For this review, use the dimensioned drawing (mm, ordinates from the lowest corner) and the shaded views. A direction names the side the tool comes from. Coordinates: 2 decimals unless noted, no trailing zeros. Order: outer loops, then holes, each group sorted by start corner. A loop starts at its lowest first (then second) coordinate and runs counter-clockwise, first axis right, second up. Notation, with made-up numbers: M -16.5,61 L -11.5,61 A23 cw -11.5,80 Z; hole C 17.25,-30.5 d1. An arc over 180 degrees is marked long. One line per item, written item: value.
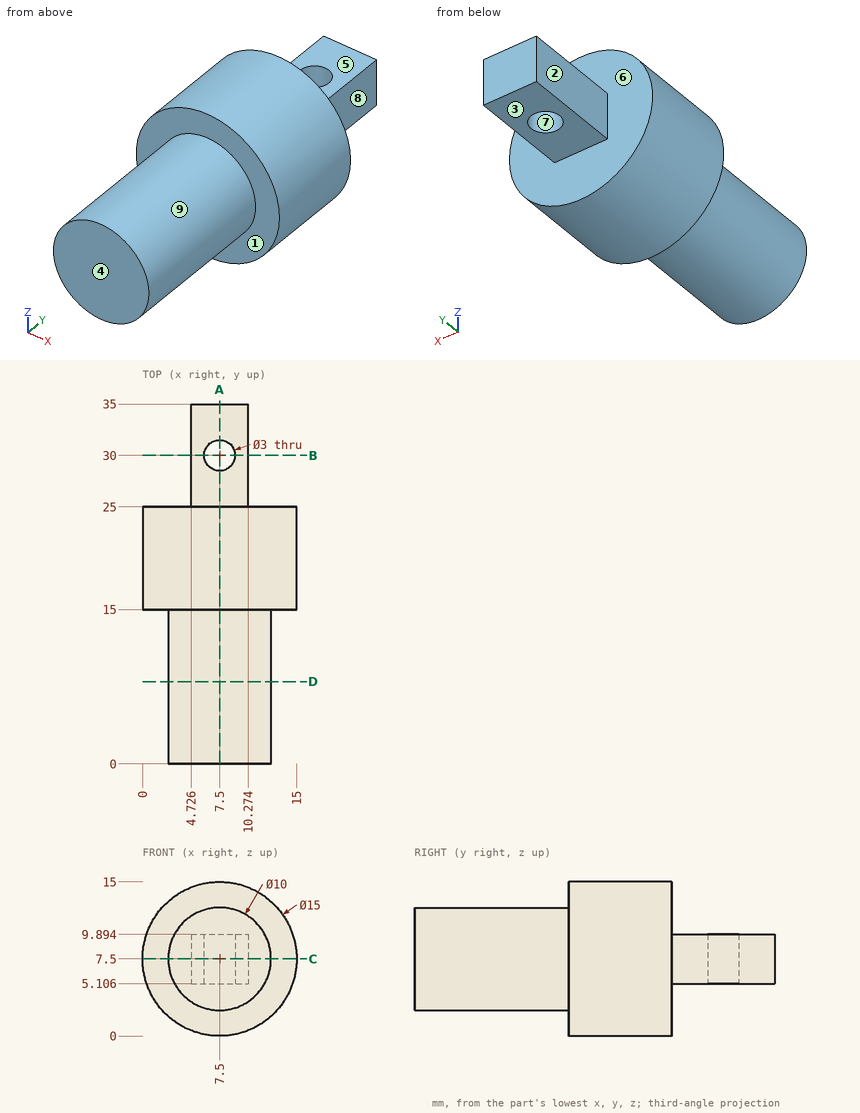
(1) We need section B-B, the plane y = 30. State the section outline as (x, z) points, plus the area to 3 significant figures.
Geometry results:
outline: M 4.73,5.11 L 6,5.11 L 6,9.89 L 4.73,9.89 Z; M 9,5.11 L 10.27,5.11 L 10.27,9.89 L 9,9.89 Z
area: 12.2 mm2
(2) We need section A-A, the plane x = 7.5. State the section outline as (y, z) points.
Geometry results:
outline: M 0,2.5 L 15,2.5 L 15,0 L 25,0 L 25,5.11 L 28.5,5.11 L 28.5,9.89 L 25,9.89 L 25,15 L 15,15 L 15,12.5 L 0,12.5 Z; M 31.5,5.11 L 35,5.11 L 35,9.89 L 31.5,9.89 Z
(3) Tool access review of the marked faces 1, 2, 3, 4 and 5: name each direction out of +Z, -Z, +X, -X, +Y, -Y from which nothing blocks a thin tool from reaching the whole face with its end or side.
Geometry results:
face 1: -Y
face 2: +Z, -Z, -X, +Y
face 3: -Z, +X, -X, +Y
face 4: +Z, -Z, +X, -X, -Y
face 5: +Z, +X, -X, +Y
(4) For L1, parallel to Y at x = 7.5, z = 7.85; L2, parallel to Y at x = 13.75, z = 6.5; L3, parallel to Z at x = 8.75, y = 31, list the stretches that pass through material, from the lowest coordinate up.
Geometry results:
L1: y = 0 to 28.5, 31.5 to 35
L2: y = 15 to 25
L3: z = 5.11 to 9.89
(5) We need section D-D, the plane y = 8. State the section outline as (x, z) points.
Geometry results:
outline: C 7.5,7.5 d10
(6) We need section C-C, the plane z = 7.5. State the section outline as (x, y) points.
Geometry results:
outline: M 0,15 L 2.5,15 L 2.5,0 L 12.5,0 L 12.5,15 L 15,15 L 15,25 L 10.27,25 L 10.27,35 L 4.73,35 L 4.73,25 L 0,25 Z; hole C 7.5,30 d3
(7) Mouldability with a two-part tool opening along X and no side actions: class the marked faces 6, 7, 8 and 9 as +X half, -X half, draft (parallel to the pull), parting line (faces both ways), or undercut.
Geometry results:
face 6: draft
face 7: undercut
face 8: +X half
face 9: parting line
(8) Insertion check: pin 1 Ø3 at (y, z) = (29.5, 6.5) entering from -X; pin 2 Ø4 at (y, z) = (14, 3) entering from -X; pin 3 Ø1.5 at (x, z) = (12, 9) entering from +Y. Each pin has a flat end and moves straight along its axis. Give the tip position at first contact, or say it passes through.
Geometry results:
pin 1: stops at x = 4.73
pin 2: stops at x = 0.53
pin 3: stops at y = 25
